```python
from build123d import *

# Parameters (mm, degrees)
SKETCH_W           = 27.75
SKETCH_H           = 13.3
PAD_DEPTH          = 1
PAD001_DEPTH       = 1.5
PAD002_START       = -0.5
SKETCH002_W        = 47.75
SKETCH002_H        = 33.3
PAD002_DEPTH       = 0.5
CHAMFER_SIZE2      = 1.49
CHAMFER_SIZE       = 1.05
CHAMFER_FACE13_W   = 33.3
CHAMFER_FACE13_H   = 47.75
CHAMFER_FACE13_W_2 = 13.3
CHAMFER_FACE13_H_2 = 27.75
POCKET_DEPTH       = 5
POCKET001_DEPTH    = 30
FILLET_R           = 0.5
SKETCH004_W        = 11.377
SKETCH004_H        = 7.673
POCKET002_DEPTH    = 1.5


with BuildPart() as part:
    # Sketch → Pad (new body)
    with BuildSketch(Plane.XY):
        with Locations((13.875, 6.65)):
            Rectangle(SKETCH_W, SKETCH_H)
    extrude(amount=PAD_DEPTH)

    # Sketch001 (on Face6 of Pad) → Pad001 (join)
    with BuildSketch(Plane.XY.offset(1)):
        with BuildLine():
            ThreePointArc((0, 13.3), (13.875, 12.3), (27.75, 13.3))
            Line((27.75, 0), (27.75, 13.3))
            ThreePointArc((27.75, 0), (13.875, 1), (0, 0))
            Line((0, 13.3), (0, 0))
        make_face()
    extrude(amount=PAD001_DEPTH)

    # Sketch002 (on Face4 of Pad001) → Pad002 (join)
    with BuildSketch(Plane(origin=(0, 0, 0), x_dir=(1, 0, 0), z_dir=(0, 0, -1)).offset(PAD002_START)):
        with Locations((13.875, -6.65)):
            Rectangle(SKETCH002_W, SKETCH002_H)
    extrude(amount=-PAD002_DEPTH)

    # Chamfer
    chamfer_edges = [part.edges().sort_by_distance(p)[0] for p in [
        (13.875, 12.3, 1),
        (13.875, 1, 1),
    ]]
    chamfer_side = part.faces().sort_by_distance((13.875, -9.417853, 1))[0]
    chamfer(chamfer_edges, length=CHAMFER_SIZE, length2=CHAMFER_SIZE2, reference=chamfer_side)

    # Chamfer Face13 → Pocket (cut)
    with BuildSketch(Plane(origin=(13.875, 6.65, 0.5), x_dir=(0, -1, 0), z_dir=(0, 0, -1))):
        Rectangle(CHAMFER_FACE13_W, CHAMFER_FACE13_H)
        Rectangle(CHAMFER_FACE13_W_2, CHAMFER_FACE13_H_2, mode=Mode.SUBTRACT)
    extrude(amount=-POCKET_DEPTH, mode=Mode.SUBTRACT)

    # Sketch003 (on Face8 of Pocket) → Pocket001 (cut)
    with BuildSketch(Plane(origin=(0, 13.3, 0), x_dir=(-1, 0, 0), z_dir=(0, 1, 0))):
        with BuildLine():
            Line((-27.75, 2.49), (-27.75, 1.99))
            ThreePointArc((0, 1.99), (-13.875, 2.49), (-27.75, 1.99))
            Line((0, 2.49), (0, 1.99))
            Line((0, 2.99), (0, 2.49))
            Line((-27.75, 2.99), (0, 2.99))
            Line((-27.75, 2.49), (-27.75, 2.99))
        make_face()
    extrude(amount=-POCKET001_DEPTH, mode=Mode.SUBTRACT)

    # Fillet
    fillet_edges = [part.edges().sort_by_distance(p)[0] for p in [
        (27.75, 13.3, 0.995),
        (27.75, 0, 0.995),
        (0, 13.3, 0.995),
        (0, 0, 0.995),
    ]]
    fillet(fillet_edges, radius=FILLET_R)

    # Sketch004 (on Face4 of Pocket) → Pocket002 (cut)
    with BuildSketch(Plane.XY.offset(2.5)):
        with Locations((13.875, 6.65)):
            Rectangle(SKETCH004_W, SKETCH004_H)
    extrude(amount=-POCKET002_DEPTH, mode=Mode.SUBTRACT)


solid = part.part
```
Geometry check sheet. Reference: the model listing, model coordinates, mm. A direction names the side the tool comes from. Give positions to 0.01 mm unless a question says otherwise; leave off trailing zeros. Use CSV: the item, a comma, the result in double quotes. Start each with the question number.
Q1. Release check for a two-part mould opening along Y. For faces 1 (the face through (0, 7, 1)), 2 (the face through (8.186, 7, 2)), 3 (the face through (14.1, 0, 0.8)) record: +Y half, -Y half, draft (parallel to the pull), parting line (faces both ways), or undercut.
Q2. Go/stop test with flat-tipped pins: pin 1 Ø4 at (x, y) = (12, 5) entering from +Z; pin 2 Ø0.7 at (x, z) = (14.5, 1.5) entering from -Y. Record where each tip stops, or that it passes through.
Q3. Access from +Z, -Z, +X, -X, +Y, -Y to the whole of each face (thin tool, end or side, straight path). Record for faces 4 (the face through (14, 7, 0)), 5 (the face through (14, 7, 1)).
Q4. Scan lines: probe 1 along Z at (x, y) = (15.75, 7.75); probe 2 along Z at (x, y) = (25.75, 8.5); probe 3 along X at (y, z) = (5, 1.35). Record each from-to range of solid material in increasing order. Write a range as from..to.
Findings below:
1,face 1,"draft"
1,face 2,"undercut"
1,face 3,"-Y half"
2,pin 1,"stops at z = 1"
2,pin 2,"stops at y = 0.05"
3,face 4,"-Z, +X, -X, +Y, -Y"
3,face 5,"+Z"
4,probe 1,"z = 0..1"
4,probe 2,"z = 0..2.12"
4,probe 3,"x = 0..8.19, 19.56..27.75"
